Autodesk Inventor part; units mm, degrees
ref_plane "YZ Plane" through (0, 0, 0) normal (1, 0, 0) x (0, 1, 0)
ref_plane "XZ Plane" through (0, 0, 0) normal (0, 1, 0) x (-1, 0, 0)
ref_plane "XY Plane" through (0, 0, 0) normal (0, 0, 1) x (1, 0, 0)
sketch "Náčrt1" plane through (0, 0, 0) normal (0, 0, 1) x (1, 0, 0)
  line L0 (-8, 0) -> (8, 0)
  line L1 (8, 0) -> (8, 27.5) construction
  line L2 (8, 27.5) -> (5.5, 27.5) construction
  line L3 (5.5, 27.5) -> (5.5, 26.5) construction
  line L4 (0.5, 21.5) -> (-0.5, 21.5) construction
  line L5 (-5.5, 26.5) -> (-5.5, 27.5) construction
  line L6 (-5.5, 27.5) -> (-8, 27.5) construction
  line L7 (-8, 27.5) -> (-8, 0) construction
  line L8 (-8, 16) -> (-6.85, 16) construction
  line L9 (-6.85, 16) -> (-6.85, 17.25) construction
  line L10 (-6.85, 17.25) -> (-5, 17.25) construction
  line L11 (-5, 17.25) -> (-5, 16) construction
  line L12 (-5, 16) -> (5, 16) construction
  line L13 (5, 16) -> (5, 14) construction
  line L14 (5, 14) -> (8, 14) construction
  arc A0 (-5.5, 26.5) -> (-0.5, 21.5) centre (-0.5, 26.5) ccw construction
  arc A1 (0.5, 21.5) -> (5.5, 26.5) centre (0.5, 26.5) ccw construction
  line L15 (5, 6) -> (5, 8)
  line L16 (5, 8) -> (10, 8)
  line L17 (10, 8) -> (10, 0)
  line L18 (10, 0) -> (8, 0)
  line L19 (-10, 6) -> (-10, 0)
  line L20 (-10, 0) -> (-8, 0)
  line L21 (-5, 6) -> (-5, 5.75)
  line L22 (-5, 5.75) -> (-6.1, 5.75)
  line L23 (-6.1, 5.75) -> (-6.1, 6)
  line L24 (-5, 6) -> (5, 6)
  line L25 (-6.1, 6) -> (-10, 6)
  point P0 (0, 0)
  point P1 (0, 0)
  point P2 (5.5, 21.5)
  point P3 (-5.5, 21.5)
  dimension "d0" = 55
  dimension "d1" = 16
  dimension "d3" = 2.5
  dimension "d4" = 6
  dimension "d5" = 32
  dimension "d6" = 28
  dimension "d7" = 10
  dimension "d8" = 13
  dimension "d9" = 34.5
  dimension "d10" = 1.85
  dimension "d18" = 11
  dimension "d24" = 43
  dimension "d27" = 5
  dimension "d31" = 16
  dimension "d32" = 2
  dimension "d33" = 2
  dimension "d34" = 1.1
  dimension "d35" = 11.5
  dimension "d36" = 12
  dimension "d37" = 20
revolve "Rotace1" add sketch "Náčrt1" angle 360 about axis through (-8, 0, 0) along (1, 0, 0)
chamfer "Zkosení1" distance 0.5 angle 45 3 edges at (10, -8, 0) (-10, -6, 0) (5, -8, 0)
hole "Díra1" at (10, 0, 0) direction (-1, 0, 0) diameter 8.4 end through all
chamfer "Zkosení3" distance 0.4 angle 45 2 edges at (-10, 0, 4.2) (10, 0, 4.2)
properties part number "DD_KVD_004_03" material "Nerezová ocel"
CAD build for the part. Positions are in the model's coordinates, mm. A direction names the side the tool comes from. Coordinates: 2 decimals unless noted, no trailing zeros. Write each loop counter-clockwise with the first axis right and the second up, starting at its lowest first coordinate (ties: lowest second). Pieces come first, ordered by that corner, then holes.
(1) 3-axis set-ups, long thin cutter, end or side, ignore diameter. For faces 5 (the face through (-8, -6, 0)), 6 (the face through (7.53, -1.73, -7.81)): which of +Z, -Z, +X, -X, +Y, -Y reach the whole face in a straight line?
(2) Two-plate mould, pull along X, no slides. Class faces 1 (the face through (10, 0, -5)), 2 (the face through (0, -6, 0)), 3 (the face through (5, 2, 6)), 4 (the face through (-5.56, -0.75, -5.7)): +X half, -X half, draft (parallel to the pull), parting line (faces both ways), or undercut.
(3) Drill centre lines: probe 1 along Z at (x, y) = (5.75, 0); probe 2 along Z at (x, y) = (-3.25, 0); probe 3 along Y at (x, z) = (-6, 1.75). Where is each one in solid material? Low to high.
(4) Cut at C-C, the plane x = 5.75. List the corners of the cut face in (y, z), and give its area (3 significant figures).
(5) Flat gauge pins, fed straight in: pin 1 (7.5 mm diameter, centred on y = -2.5, z = -2.5, fed in from -X); pin 2 (3 mm diameter, centred on x = -7.5, z = -4.5, fed in from +Y); pin 3 (1.5 mm diameter, centred on x = 0, z = 1, fed in from +Y); pin 4 (3 mm diameter, centred on x = -6, z = 1.5, fed in from -Y). Where does each tip first touch, or does it go through?
(6) Cut at B-B, the plane x = 0.75. List the corners of the cut face in (y, z), and give its area (3 significant figures).
Geometry says:
1. face 5: -X
1. face 6: +X, -X
2. face 1: +X half
2. face 2: draft
2. face 3: -X half
2. face 4: undercut
3. probe 1: z = -8 to -4.2, 4.2 to 8
3. probe 2: z = -6 to -4.2, 4.2 to 6
3. probe 3: y = -5.48 to -3.82, 3.82 to 5.48
4. outline: circle Ø16 at (0, 0); hole circle Ø8.4 at (0, 0)
4. area: 146 mm2
5. pin 1: stops at x = -10
5. pin 2: stops at y = 5.2
5. pin 3: stops at y = 5.99
5. pin 4: stops at y = -6
6. outline: circle Ø12 at (0, 0); hole circle Ø8.4 at (0, 0)
6. area: 57.7 mm2
